Autodesk Inventor part; units mm, degrees
ref_plane "YZ Plane" through (0, 0, 0) normal (1, 0, 0) x (0, 1, 0)
ref_plane "XZ Plane" through (0, 0, 0) normal (0, 1, 0) x (-1, 0, 0)
ref_plane "XY Plane" through (0, 0, 0) normal (0, 0, 1) x (1, 0, 0)
sketch "Szkic1" plane through (0, 0, 0) normal (0, 1, 0) x (-1, 0, 0)
  line L0 (12, 18) -> (-12, 18)
  line L1 (-12, 18) -> (-12, -18)
  line L2 (-12, -18) -> (12, -18)
  line L3 (12, -18) -> (12, 18)
  line L4 (12, 18) -> (-12, -18) construction
  line L5 (-12, 18) -> (12, -18) construction
  line L6 (15, 21) -> (-15, 21)
  line L7 (-15, 21) -> (-15, -21)
  line L8 (-15, -21) -> (15, -21)
  line L9 (15, -21) -> (15, 21)
  line L10 (15, 21) -> (-15, -21) construction
  line L11 (-15, 21) -> (15, -21) construction
  line L12 (9, 15) -> (-9, 15)
  line L13 (-9, 15) -> (-9, -15)
  line L14 (-9, -15) -> (9, -15)
  line L15 (9, -15) -> (9, 15)
  line L16 (9, 15) -> (-9, -15) construction
  line L17 (-9, 15) -> (9, -15) construction
  point P0 (0, 0)
  dimension "d0" = 24
  dimension "d1" = 36
  dimension "d2" = 42
  dimension "d3" = 30
  dimension "d4" = 18
  dimension "d5" = 30
extrude "Wyciągnięcie proste1" add sketch "Szkic1" along normal blind 3 contours L3 L2 L1 L0
extrude "Wyciągnięcie proste2" add sketch "Szkic1" along normal blind 8 contours L9 L8 L7 L6
sketch "Szkic2" plane through (0, 8, 0) normal (0, 1, 0) x (1, 0, 0)
  line L0 (-15, 21) -> (-15, -21)
  line L1 (-12, -18) -> (12, -18)
  line L2 (-15, -21) -> (-4, -21)
  line L3 (-4, -21) -> (-4, -18)
  line L4 (-4, -18) -> (-15, -18)
  line L5 (-15, -18) -> (-15, -21)
  line L6 (-12, -18) -> (-15, -18)
  line L7 (-15, -18) -> (-15, -10)
  line L8 (-15, -10) -> (-12, -10)
  line L9 (-12, -10) -> (-12, -18)
  line L10 (-15, -21) -> (-15, -10)
  line L11 (0, 0) -> (-18.1992, 0)
  line L12 (-15, 21) -> (-4, 21)
  line L13 (-4, 21) -> (-4, 18)
  line L14 (-4, 18) -> (-15, 18)
  line L15 (-15, 10) -> (-12, 10)
  line L16 (-12, 10) -> (-12, 18)
  line L17 (4, 18) -> (15, 18)
  line L18 (4, 21) -> (4, 18)
  line L19 (15, 21) -> (4, 21)
  line L20 (15, 21) -> (15, 10)
  line L21 (15, 10) -> (12, 10)
  line L22 (12, 10) -> (12, 18)
  line L23 (12, -10) -> (12, -18)
  line L24 (15, -10) -> (12, -10)
  line L25 (4, -18) -> (15, -18)
  line L26 (15, -21) -> (4, -21)
  line L27 (4, -21) -> (4, -18)
  line L28 (15, -21) -> (15, 21)
  line L29 (15, -21) -> (15, -10)
  point P0 (-4, -19.5)
  point P1 (4, 19.5)
  dimension "d10" = 11
  dimension "d11" = 8
  dimension "d12" = 18.1992
  dimension "d15" = 360
extrude "Wyciągnięcie proste3" add sketch "Szkic2" along normal blind 75
sketch "Szkic3" plane through (-4, 8, 21) normal (1, 0, 0) x (0, 0, -1)
  line L0 (0, 75) -> (3, 75)
  line L1 (3, -5) -> (3, 75)
  line L2 (0, 75) -> (3, 75)
  line L3 (3, 75) -> (3, 69)
  line L4 (3, 69) -> (0, 69)
  line L5 (0, 69) -> (0, 75)
  line L6 (21, 73.1209) -> (21, -14.9491)
  line L7 (0, -8) -> (0, 75)
  line L8 (42, 75) -> (39, 75)
  line L9 (39, -5) -> (39, 75)
  line L10 (39, 69) -> (42, 69)
  line L11 (42, 69) -> (42, 75)
  point P0 (21, -8)
  dimension "d19" = 6
  dimension "d20" = 88.0699
  dimension "d21" = 21
extrude "Wyciągnięcie proste4" add sketch "Szkic3" along normal blind 9
sketch "Szkic7" plane through (-15, 0, 21) normal (0, 0, 1) x (1, 0, 0)
  line L0 (27, 83) -> (3, 83)
  line L1 (12, 83) -> (18, 83)
  line L2 (18, 83) -> (18, 79)
  line L3 (18, 79) -> (12, 79)
  line L4 (12, 79) -> (12, 83)
  line L5 (19, 8) -> (19, 77)
  point P0 (15, 0)
  point P1 (18, 81)
  dimension "d29" = 6
  dimension "d30" = 1
  dimension "d31" = 4
extrude "Wyciągnięcie proste6" add sketch "Szkic7" along normal blind 6.25
mirror "Odbij1" about plane through (0, 0, 0) normal (0, 0, 1) of "Wyciągnięcie proste6"
sketch "Szkic8" plane through (0, 83, 0) normal (0, 1, 0) x (1, 0, 0)
  line L0 (3, -27.25) -> (-3, -27.25)
  line L1 (-3, -21) -> (-3, -27.25)
  point P0 (0, 0)
  point P1 (0, -24.25)
  dimension "d34" = 3
  dimension "d35" = 3
hole "Otwór1" at (0, 83, 24.25) direction (0, -1, 0) diameter 3.2 end through all
mirror "Odbij2" about plane through (0, 0, 0) normal (0, 0, 1) of "Otwór1"
properties part number "mocowanie-bateria"
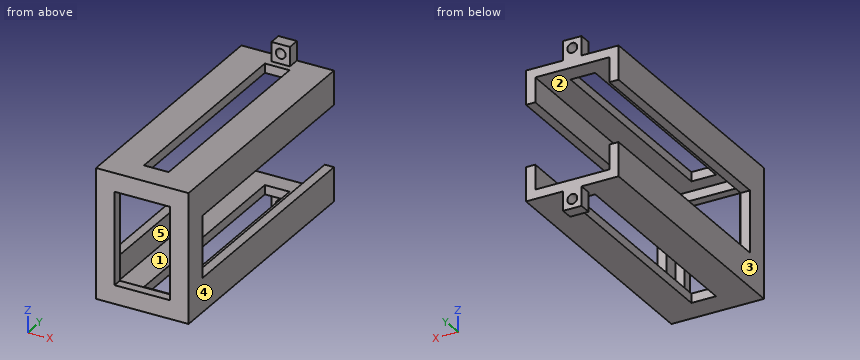
Here's how the part is built. I have some questions about the finished solid (model axes, mm). Face numbers are marked on the shaded views. A direction names the side the tool comes from. Give positions to 0.01 mm unless a question says otherwise; leave off trailing zeros. Write each loop counter-clockwise with the first axis right and the second up, starting at its lowest first coordinate (ties: lowest second). Pieces come first, ordered by that corner, then holes. Notation, with made-up numbers: M 11,56.5 L 69,56.5 A12 ccw 69,69.5 Z; hole C 44,74.25 d7. An arc over 180 degrees is marked long. Put each result on its own line as item: value. Start each with the question number.
Item 1: Will these pins go through, and if not, where does the flat tip stop? pin 1 (6 mm diameter, centred on x = -3, y = 57, fed in from -Z); pin 2 (1.8 mm diameter, centred on x = -0.5, z = 25.5, fed in from -Y); pin 3 (0.9 mm diameter, centred on x = -14, y = 44, fed in from +Z); pin 4 (10 mm diameter, centred on x = 11.5, z = 20.5, fed in from -Y).
Item 2: If we section it at D-D, the plane x = 0: Count the separate pieces of the cut face and the enclosed holes in it, then the cut area to 3 significant figures.
Item 3: If we section it at C-C, the plane z = 24.25: Write out the boundary of the cut face in (x, y).
Item 4: On a 3-axis mill with a long thin cutter (end or side, diameter ignored), from which of +Z, -Z, +X, -X, +Y, -Y can I reach the whole of each face in a straight line? I mean the marked faces 4 and 5. Say none if no direction works.
Item 5: Thinking about a two-plate mould opening in Z: for the marked faces 1, 2 and 3, which applies, +Z half, -Z half, draft (parallel to the pull), parting line (faces both ways), or undercut?
Item 6: If we section it at B-B, the plane y = 18: Write out the boundary of the cut face in (x, z), then the cut area to 3 significant figures.
Item 7: I need wall thicknesses on L1, parallel to Z at x = 0, y = 81.55; L2, parallel to X at y = 82.1, z = 24.25; L3, parallel to X at y = 6, z = 12. Which ranges of each line are inside material? Lowest first, please. Write a range as from..to.
Item 8: If we section it at A-A, the plane x = 7: Write out the boundary of the cut face in (y, z), then the cut area to 3 significant figures.
Values:
1. pin 1: z = -21
1. pin 2: y = 79
1. pin 3: z = 21
1. pin 4: y = 0
2. separate pieces: 6
2. enclosed holes: 0
2. area: 126 mm²
3. outline: M -3,79 L -1.6,79 L -1.6,83 L -3,83 Z; M 1.6,79 L 3,79 L 3,83 L 1.6,83 Z
4. face 4: +Z, -Z, +X, +Y, -Y
4. face 5: +Y
5. face 1: undercut
5. face 2: undercut
5. face 3: draft
6. outline: M -15,-21 L -4,-21 L -4,-18 L -12,-18 L -12,-10 L -15,-10 Z; M -15,10 L -12,10 L -12,18 L -4,18 L -4,21 L -15,21 Z; M 4,-21 L 15,-21 L 15,-10 L 12,-10 L 12,-18 L 4,-18 Z; M 4,18 L 12,18 L 12,10 L 15,10 L 15,21 L 4,21 Z
6. area: 228 mm²
7. L1: -27.25..-25.85, -22.65..-18, 18..22.65, 25.85..27.25
7. L2: -3..-1.6, 1.6..3
7. L3: -15..-12, 12..15
8. outline: M 0,-21 L 83,-21 L 83,-18 L 3,-18 L 3,-15 L 0,-15 Z; M 0,15 L 3,15 L 3,18 L 83,18 L 83,21 L 0,21 Z
8. area: 516 mm²
